Geometry check sheet. Reference: the model listing, model coordinates, mm. A direction names the side the tool comes from. Give positions to 0.01 mm unless a question says otherwise; leave off trailing zeros. Order: outer loops, then holes, each group sorted by start corner. A loop starts at its lowest first (then second) coordinate and runs counter-clockwise, first axis right, second up. Notation, with made-up numbers: (29, 3) - (72, 3) arc R21 ccw to (72, 14) - close; hole circle Ø3 at (30, -2). An arc over 180 degrees is marked (long way). Put each result on its own line as item: value. Start each with the question number.
```python
from build123d import *


with BuildPart() as f1:
    # F0 (on Front) → F1 (revolve)
    with BuildSketch(Plane.XZ):
        with BuildLine():
            Line((3.81, 0), (3.81, 7.62))
            add(Edge.make_bspline(
                [(3.81, 7.62), (0.889, 7.62), (0.889, 0)],
                knots=[0, 0, 0, 1.5707963268, 1.5707963268, 1.5707963268], degree=2, weights=[1, 0.7071067812, 1]))
            Line((0.889, 0), (3.81, 0))
        make_face()
        Polygon((7.3152, 0), (3.81, 0), (0.889, 0), (0.889, -1.27), (6.0452, -1.27), (6.0452, -5.334), (7.3152, -5.334), align=None)
        Polygon((7.3152, -5.588), (7.3152, -5.334), (6.0452, -5.334), (5.5372, -5.334), (5.5372, -5.588), align=None)
    revolve(axis=Axis((0, 0, 8.5612153634), (0, 0, 1)))


solid = f1.part
```
Item 1: Cross-section at A-A (z = -3). Enter the section's corners in (x, y).
Item 2: Gauge pin test, flat ends, axial feed: pin 1 Ø2.5 at (x, y) = (0, 0) entering from -Z; pin 2 Ø1.5 at (y, z) = (4, -2) entering from +X; pin 3 Ø1 at (y, z) = (6, 4) entering from -X. Record the tip position at first contact, or that the pin passes through.
Item 3: Thickness scan on line 1 along Z through (x, y) = (-5.5, 1.5); line 2 along Y through (x, z) = (0, -0.75); line 3 along Y through (x, z) = (-5.5, -2.75). Record the ranges inside material, lowest first.
Item 4: Cross-section at B-B (x = -4.5). Enter the section's corners in (y, z), and give its area (3 significant figures).
Item 5: Release check for a two-part mould opening along Y. For faces 3 (the face through (3, -3, 0)), 4 (the face through (-0.83, -3.72, 3.86)), 5 (the face through (0.1, -1.3, -1.27)) record: +Y half, -Y half, draft (parallel to the pull), parting line (faces both ways), or undercut.
Item 6: Set-up check for faces 1 (the face through (-3, 5, -5.588)), 2 (the face through (-1.31, -5.9, -3.33)): record each of +Z, -Z, +X, -X, +Y, -Y from which the full face is reachable in a straight line by a thin tool's end or side.
Recorded:
1. outline: circle Ø14.63 at (0, 0); hole circle Ø12.09 at (0, 0)
2. pin 1: stops at z = -1.27
2. pin 2: stops at x = 6.55
2. pin 3: passes through
3. line 1: z = -5.59 to -5.33, -1.27 to 0
3. line 2: y = -7.32 to -0.89, 0.89 to 7.32
3. line 3: y = -4.82 to -2.51, 2.51 to 4.82
4. outline: (-5.77, -5.59) - (-3.23, -5.59) - (-3.23, -5.33) - (-4.04, -5.33) - (-4.04, -1.27) - (4.04, -1.27) - (4.04, -5.33) - (3.23, -5.33) - (3.23, -5.59) - (5.77, -5.59) - (5.77, 0) - (-5.77, 0) - close
4. area: 30.0 mm^2
5. face 3: draft
5. face 4: parting line
5. face 5: undercut
6. face 1: -Z, +X, -X, +Y, -Y
6. face 2: none
